For this review, use the dimensioned drawing (mm, ordinates from the lowest corner) and the shaded views. A direction names the side the tool comes from. Coordinates: 2 decimals unless noted, no trailing zeros. Loops run counter-clockwise (first coordinate to the right, second up) from the corner with the lowest first, then second, coordinate; pieces in that order, holes last. Notation, with made-up numbers: (-35, -15.5) - (3, -15.5) arc R23 ccw to (3, 22.5) - close; hole circle Ø2 at (-16.5, 81). An arc over 180 degrees is marked (long way). Use a Markdown table: item, result. Add a question column.
1) Add section C-C, the plane x = 24. Give the boundary of the cut face in (y, z).
2) Add section A-A, the plane z = 44.5. Give the boundary of the cut face in (x, y).
3) To check wall thickness, follow L1, parallel to X at y = 10.5, z = 40; L2, parallel to Z at x = 22, y = 11.75. State the ranges of each line that lie inside material, in increasing order. Write a range as [from, to].
4) For the marked faces 1 and 2, list the 3-axis set-ups (+Z, -Z, +X, -X, +Y, -Y) from which the entire face can be reached by the end or side of a thin tool; tool diameter is ignored.
5) Add section B-B, the plane y = 7.75. Give the boundary of the cut face in (x, z).
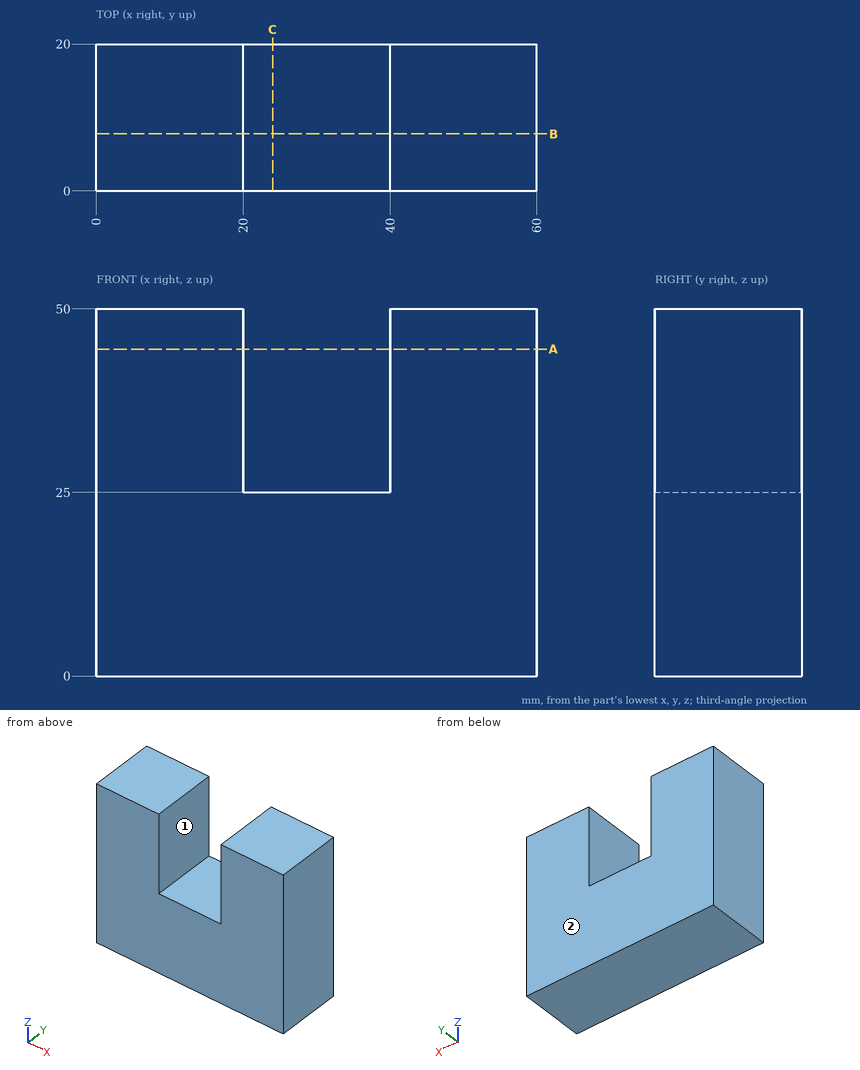
From the geometry:
| question | item | result |
|---|---|---|
| 1 | outline | (0, 0) - (20, 0) - (20, 25) - (0, 25) - close |
| 2 | outline | (0, 0) - (20, 0) - (20, 20) - (0, 20) - close; (40, 0) - (60, 0) - (60, 20) - (40, 20) - close |
| 3 | L1 | x = [0, 20], [40, 60] |
| 3 | L2 | z = [0, 25] |
| 4 | face 1 | +Z, +Y, -Y |
| 4 | face 2 | +Z, -Z, +X, -X, +Y |
| 5 | outline | (0, 0) - (60, 0) - (60, 50) - (40, 50) - (40, 25) - (20, 25) - (20, 50) - (0, 50) - close |
